CAD build for the part. Positions are in the model's coordinates, mm. Face numbers are marked on the shaded views. Round coordinates to 2 decimals unless told otherwise and drop trailing zeros. Order: outer loops, then holes, each group sorted by start corner. A loop starts at its lowest first (then second) coordinate and runs counter-clockwise, first axis right, second up. Notation, with made-up numbers: (21.5, -1.5) - (57.5, -1.5) arc R20 cw to (57.5, 31.5) - close; hole circle Ø9 at (75.25, -5). An arc over 180 degrees is marked (long way). Write item = value, one per line.
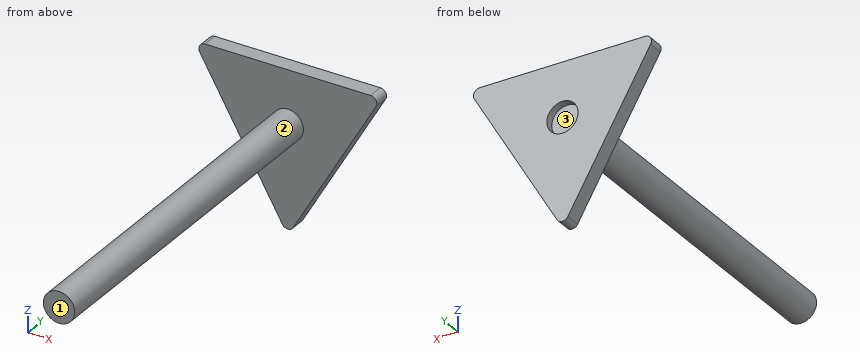
from build123d import *

# Parameters (mm, degrees)
F0_R     = 12.7
F1_DEPTH = 6.35
F2_R     = 5.08
F3_DEPTH = 304.8


with BuildPart() as f1:
    # F0 (on Front) → F1 (new body, symmetric)
    with BuildSketch(Plane.XZ):
        Polygon((76.2, 43.994091), (-76.2, 43.994091), (0, -87.988181), align=None)
        Circle(F0_R, mode=Mode.SUBTRACT)
    extrude(amount=F1_DEPTH, both=True)

    # F2
    f2_edges = [f1.edges().sort_by_distance(p)[0] for p in [
        (0, 0, -87.988181),
        (76.2, 0, 43.994091),
        (-76.2, 0, 43.994091),
    ]]
    fillet(f2_edges, radius=F2_R)

    # F0 (on Front) → F3 (join)
    with BuildSketch(Plane.XZ):
        Circle(F0_R)
    extrude(amount=F3_DEPTH)


solid = f1.part
(1) Band-saw the part on D-D on x = 25. List the corners of the cut face in (y, z).
Solved:
outline = (-6.35, -44.69) - (6.35, -44.69) - (6.35, 43.99) - (-6.35, 43.99) - close
(2) Pull direction X, two halves, no side cores. Call the marked faces 1, 2 and 3: released by +X, released by -X, zero draft, split by the parting line, or undercut.
Solved:
face_1 = zero draft
face_2 = split by the parting line
face_3 = undercut
(3) Band-saw the part on B-B on z = 0. List the corners of the cut face in (x, y), plus the area to 3 significant figures.
Solved:
outline = (-50.8, -6.35) - (-12.7, -6.35) - (-12.7, -304.8) - (12.7, -304.8) - (12.7, -6.35) - (50.8, -6.35) - (50.8, 6.35) - (12.7, 6.35) - (12.7, 0) - (-12.7, 0) - (-12.7, 6.35) - (-50.8, 6.35) - close
area = 8,710 mm²
(4) Band-saw the part on A-A on x = 0. List the corners of the cut face in (y, z).
Solved:
outline = (-304.8, -12.7) - (-6.35, -12.7) - (-6.35, -82.91) - (6.35, -82.91) - (6.35, -12.7) - (0, -12.7) - (0, 12.7) - (6.35, 12.7) - (6.35, 43.99) - (-6.35, 43.99) - (-6.35, 12.7) - (-304.8, 12.7) - close
(5) Band-saw the part on C-C on y = -65. List the corners of the cut face in (x, z).
Solved:
outline = circle Ø25.4 at (0, 0)
(6) Drop flat-ended pins along their axis: pin 1 (6 mm diameter, centred on x = -11.5, y = -77.5, fed in from -Z); pin 2 (7.5 mm diameter, centred on x = 4.5, z = 6, fed in from +Y). Give the stop position or say it passes through.
Solved:
pin_1 = -9.44
pin_2 = 0
(7) Probe line 1 along Y through (x, z) = (45, 13.5); line 2 along Y through (x, z) = (-5, -4); line 3 along Z through (x, y) = (5.5, -73). List the from-to ranges inside material, lowest first.
Solved:
line_1 = -6.35 to 6.35
line_2 = -304.8 to 0
line_3 = -11.45 to 11.45
